```python
from build123d import *

# Parameters (mm, degrees)
BOSS_EXTRUDE1_DEPTH = 2000
CUT_EXTRUDE1_REACH  = 2423.496
SKETCH3_W           = 311
SKETCH3_H           = 115
SKETCH2_W           = 1960
SKETCH2_H           = 178.8
CUT_EXTRUDE2_DEPTH  = 310
FILLET2_R           = 10
FILLET3_R           = 2


with BuildPart() as part:
    # Sketch1 → Boss-Extrude1 (new body)
    with BuildSketch(Plane.XY):
        Polygon((0, 0), (735, 0), (735, 1150.4), (667.5, 1150.4), (667.5, 218.8), (0, 218.8), align=None)
    extrude(amount=BOSS_EXTRUDE1_DEPTH)

    # Sketch3 → Cut-Extrude1 (cut, up to next)
    with BuildSketch(Plane(origin=(0, 0, 0), x_dir=(-1, 0, 0), z_dir=(0, 0, -1)), mode=Mode.PRIVATE) as cut_extrude1_sk1:
        with Locations((-579.5, 57.5)):
            Rectangle(SKETCH3_W, SKETCH3_H)
    cut_extrude1_tool1 = extrude(cut_extrude1_sk1.sketch, amount=-CUT_EXTRUDE1_REACH, mode=Mode.PRIVATE) & part.part
    add(cut_extrude1_tool1.solids().sort_by_distance((579.5, 57.5, 0))[0], mode=Mode.SUBTRACT)

    # Sketch2 → Cut-Extrude2 (cut)
    with BuildSketch(Plane.ZY):
        with Locations((1000, 109.4)):
            Rectangle(SKETCH2_W, SKETCH2_H)
    extrude(amount=-CUT_EXTRUDE2_DEPTH, mode=Mode.SUBTRACT)

    # Fillet2
    fillet2_edges = [part.edges().sort_by_distance(p)[0] for p in [
        (735, 1150.4, 1000),
        (0, 0, 1000),
        (0, 218.8, 1000),
        (667.5, 218.8, 1000),
        (667.5, 1150.4, 1000),
        (333.75, 218.8, 2000),
        (0, 109.4, 2000),
        (735, 632.7, 0),
        (212, 0, 2000),
        (735, 632.7, 2000),
        (579.5, 115, 2000),
        (735, 115, 1000),
        (424, 57.5, 2000),
        (424, 0, 1000),
        (424, 57.5, 0),
        (579.5, 115, 0),
        (701.25, 1150.4, 2000),
        (212, 0, 0),
        (0, 109.4, 0),
        (333.75, 218.8, 0),
        (667.5, 684.6, 0),
        (701.25, 1150.4, 0),
        (667.5, 684.6, 2000),
    ]]
    fillet(fillet2_edges, radius=FILLET2_R)

    # Fillet3
    fillet3_edges = [part.edges().sort_by_distance(p)[0] for p in [
        (155, 198.8, 1980),
        (155, 20, 1980),
        (155, 20, 20),
        (155, 198.8, 20),
        (0, 109.4, 1980),
        (0, 198.8, 1000),
        (0, 109.4, 20),
        (0, 20, 1000),
    ]]
    fillet(fillet3_edges, radius=FILLET3_R)


solid = part.part
```
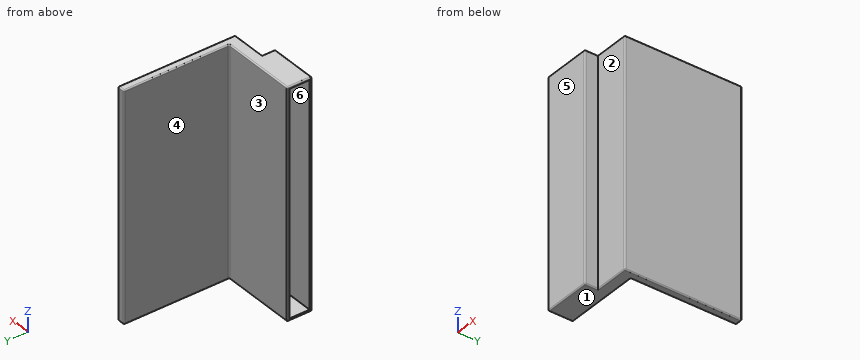
Input: part model. Units: mm. Frame: model coordinates. Face numbers are marked on the shaded views. A direction names the side the tool comes from. Give positions to 0.01 mm unless a question says otherwise; leave off trailing zeros. Order: outer loops, then holes, each group sorted by start corner. A loop starts at its lowest first (then second) coordinate and runs counter-clockwise, first axis right, second up. Notation, with made-up numbers: M 12,-19 L 43,-19 A21 cw 43,13 Z; hole C 88.5,54.5 d5. An arc over 180 degrees is marked long. One line per question, with ' | ' between items.
1) Contact query for flat-ended pins moving along their axis: P1, Ø12, axis at x = 585.5, z = 940.5, coming from the +Y side; P2, Ø1.5, axis at x = 503.5, z = 346, coming from the -Y side; P3, Ø12, axis at y = 631, z = 700, coming from the -X side. Output: stop coordinate, or through.
Filled in:
P1: stops at y = 218.8 | P2: stops at y = 115 | P3: stops at x = 667.5
2) Section B-B on z = 231.5. Output: boundary loops of the cut face in (x, y), and give its area (3 significant figures).
Filled in:
outline: M 0,10 A10 ccw 10,0 L 414,0 A10 ccw 424,10 L 424,115 L 725,115 A10 ccw 735,125 L 735,1140.4 A10 ccw 725,1150.4 L 677.5,1150.4 A10 ccw 667.5,1140.4 L 667.5,228.8 A10 cw 657.5,218.8 L 10,218.8 A10 ccw 0,208.8 L 0,200.8 A2 ccw 2,198.8 L 310,198.8 L 310,20 L 2,20 A2 ccw 0,18 Z | area: 132,000 mm2
3) Section C-C on y = 745. Output: boundary loops of the cut face in (x, z), and give its area (3 significant figures).
Filled in:
outline: M 667.5,10 A10 ccw 677.5,0 L 725,0 A10 ccw 735,10 L 735,1990 A10 ccw 725,2000 L 677.5,2000 A10 ccw 667.5,1990 Z | area: 135,000 mm2
4) Draft query along Y for the marked faces 3, 4, 5 and 6. Return one class per face: pulls with the +Y half, pulls with the -Y half, needs draft (parallel to the pull), parting line crosses it, or undercut.
Filled in:
face 3: pulls with the +Y half | face 4: needs draft | face 5: pulls with the -Y half | face 6: undercut
5) Section D-D on x = 380.5. Output: boundary loops of the cut face in (y, z).
Filled in:
outline: M 0,10 A10 ccw 10,0 L 208.8,0 A10 ccw 218.8,10 L 218.8,1990 A10 ccw 208.8,2000 L 10,2000 A10 ccw 0,1990 Z
6) Section A-A on x = 232. Output: boundary loops of the cut face in (y, z).
Filled in:
outline: M 0,10 A10 ccw 10,0 L 208.8,0 A10 ccw 218.8,10 L 218.8,1990 A10 ccw 208.8,2000 L 10,2000 A10 ccw 0,1990 Z; hole M 20,22 A2 ccw 22,20 L 196.8,20 A2 ccw 198.8,22 L 198.8,1978 A2 ccw 196.8,1980 L 22,1980 A2 ccw 20,1978 Z
7) Access query for the marked faces 1 and 2. Directions: +Z, -Z, +X, -X, +Y, -Y. A direction counts if a zero-diameter tool reaches every point of the face in a straight line with its end or side. Return the directions, or none.
Filled in:
face 1: -Z, +X, -X, +Y, -Y | face 2: +Z, -Z, +X, -Y
8) Ray query, L1, parallel to Y at x = 49, z = 1179; L2, parallel to Y at x = 379, z = 1064.5; L3, parallel to X at y = 460, z = 265. Return the intervals inside material, ascending.
Filled in:
L1: y = 0 to 20, 198.8 to 218.8 | L2: y = 0 to 218.8 | L3: x = 667.5 to 735
